Check sheet for the drawn part. Datum: minimum x, y, z corner. Units: mm. A direction names the side the tool comes from. Give positions to 0.01 mm unless a question says otherwise; leave off trailing zeros. Order: outer loops, then holes, each group sorted by start corner. A loop starts at its lowest first (then second) coordinate and runs counter-clockwise, first axis right, second up. Notation, with made-up numbers: (15, 55) -> (27, 55) arc R18 cw to (27, 61) -> close; hole circle Ø7 at (83, 27). An arc over 180 degrees is marked (long way). Answer in a Markdown table with one row per item. Add a question column.
(1) Cross-section at A-A (y = 13). Record the cut outline in (x, z) (1 decimal).
(2) Release check for a two-part mould opening along X. For the marked faces 1, 2 and 3 record: released by +X, released by -X, zero draft, split by the parting line, or undercut.
(3) Go/stop test with flat-tipped pins: pin 1 (8 mm diameter, centred on y = 42.5, z = 7.5, fed in from -X); pin 2 (3 mm diameter, centred on x = 3.5, y = 51.5, fed in from +Z) (3 decimals); pin 3 (10 mm diameter, centred on x = 20.5, z = 13.5, fed in from +Y) (3 decimals). Record where each tip stops, or that it passes through.
(4) Thickness scan on L1, parallel to X at y = 79, z = 13 (1 decimal); L2, parallel to Y at x = 20.5, z = 10.5 (1 decimal); L3, parallel to Z at x = 48.5, y = 75 (1 decimal). Record the ranges inside material, lowest first. Write a range as [from, to].
(5) Set-up check for the marked faces 4 and 5: record each of +Z, -Z, +X, -X, +Y, -Y from which the full face is reachable in a straight line by a thin tool's end or side.
(6) Cross-section at B-B (z = 9.25). State how many separate pieces and enclosed holes the cut face has, then the cut area to 3 significant figures.
(7) Cross-section at C-C (y = 82). Record the cut outline in (x, z) (1 decimal).
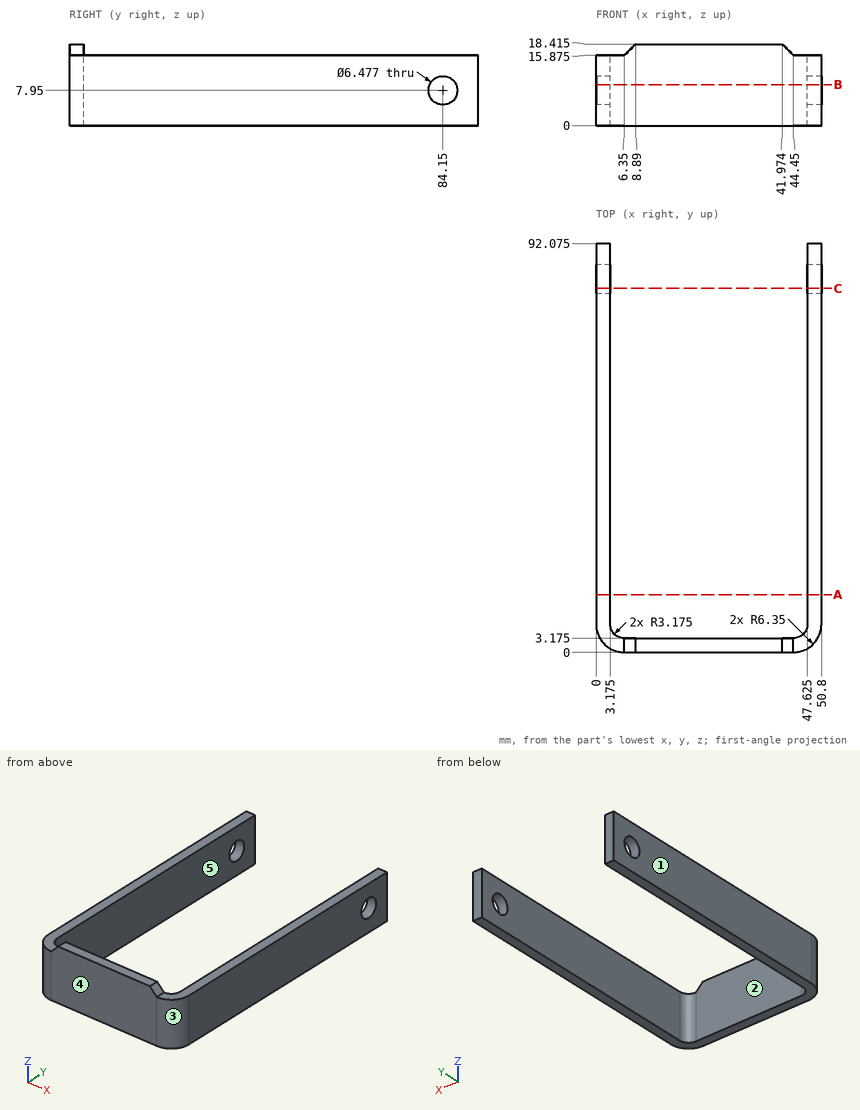
Answer below:
| question | item | result |
|---|---|---|
| 1 | outline | (0, 0) -> (3.2, 0) -> (3.2, 15.9) -> (0, 15.9) -> close; (47.6, 0) -> (50.8, 0) -> (50.8, 15.9) -> (47.6, 15.9) -> close |
| 2 | face 1 | released by -X |
| 2 | face 2 | undercut |
| 2 | face 3 | released by +X |
| 3 | pin 1 | stops at x = 0 |
| 3 | pin 2 | stops at z = 15.875 |
| 3 | pin 3 | stops at y = 3.175 |
| 4 | L1 | x = [0, 3.2], [47.6, 50.8] |
| 4 | L2 | y = [0, 3.2] |
| 4 | L3 | z = [0, 15.9] |
| 5 | face 4 | +Z, -Z, +X, -X, -Y |
| 5 | face 5 | +Z, -Z, +Y |
| 6 | separate pieces | 3 |
| 6 | enclosed holes | 0 |
| 6 | area | 675 mm² |
| 7 | outline | (0, 0) -> (3.2, 0) -> (3.2, 5.5) -> (0, 5.5) -> close; (0, 10.4) -> (3.2, 10.4) -> (3.2, 15.9) -> (0, 15.9) -> close; (47.6, 0) -> (50.8, 0) -> (50.8, 5.5) -> (47.6, 5.5) -> close; (47.6, 10.4) -> (50.8, 10.4) -> (50.8, 15.9) -> (47.6, 15.9) -> close |
